Source: CAD feature listing. Evaluate the final solid. Frame: model axes, mm. Face numbers are marked on the shaded views. A direction names the side the tool comes from. Round coordinates to 2 decimals unless told otherwise and drop trailing zeros. Loops run counter-clockwise (first coordinate to the right, second up) from the corner with the lowest first, then second, coordinate; pieces in that order, holes last. Notation, with made-up numbers: (-30, 22.5) - (17, 22.5) arc R26 ccw to (17, 52.5) - close; hole circle Ø11 at (5.25, 45). An arc over 180 degrees is marked (long way). Use CSV: the item, a comma, the result in double quotes. Start each with the question number.
from build123d import *

# Parameters (mm, degrees)
BOSS_EXTRUDE1_DEPTH = 2
BOSS_EXTRUDE2_DEPTH = 3.2
SKETCH3_OUTSIDE_W   = 10.04
SKETCH3_OUTSIDE_H   = 5.89
CUT_EXTRUDE1_DEPTH  = 4.8
SKETCH4_W           = 1
SKETCH4_H           = 0.3
CUT_EXTRUDE3_DEPTH  = 2.3
CUT_EXTRUDE6_DEPTH  = 7.038418667
SKETCH6_W           = 0.5
SKETCH6_H           = 0.5
CUT_EXTRUDE7_DEPTH  = 2
SKETCH7_W           = 0.5
SKETCH7_H           = 0.8
CUT_EXTRUDE8_DEPTH  = 7
SKETCH8_W           = 6
SKETCH8_H           = 1
CUT_EXTRUDE9_DEPTH  = 0.5


with BuildPart() as part:
    # Sketch1 → Boss-Extrude1 (new body)
    with BuildSketch(Plane.XY):
        with BuildLine():
            Line((-2.7, 1.5), (2.7, 1.5))
            ThreePointArc((2.7, 1.5), (2.912132034, 1.412132034), (3, 1.2))
            Line((3, 1.2), (3, 0))
            Line((3, 0), (-3, 0))
            Line((-3, 0), (-3, 1.2))
            ThreePointArc((-3, 1.2), (-2.912132034, 1.412132034), (-2.7, 1.5))
        make_face()
    extrude(amount=BOSS_EXTRUDE1_DEPTH)

    # Sketch2 → Boss-Extrude2 (add, symmetric)
    with BuildSketch(Plane(origin=(0, 0, 0), x_dir=(0, 0, -1), z_dir=(1, 0, 0))):
        with BuildLine():
            Line((0, 2.25), (-4.2, 2.25))
            ThreePointArc((-4.2, 2.25), (-4.6, 1.85), (-4.2, 1.45))
            Line((-4.2, 1.45), (0, 1.45))
            Line((0, 1.45), (0, 2.25))
        make_face()
    extrude(amount=BOSS_EXTRUDE2_DEPTH, both=True)

    # Sketch3 outside → Cut-Extrude1 (cut)
    with BuildSketch(Plane.XY.offset(2)):
        with Locations((0, 1.125)):
            Rectangle(SKETCH3_OUTSIDE_W, SKETCH3_OUTSIDE_H)
        with BuildLine():
            Line((-2, 2.2), (2, 2.2))
            ThreePointArc((2, 2.2), (2.212132034, 2.112132034), (2.3, 1.9))
            Line((2.3, 1.9), (2.3, 1.1))
            Line((2.3, 1.1), (1.8, 0.6))
            Line((1.8, 0.6), (-1.8, 0.6))
            Line((-1.8, 0.6), (-2.3, 1.1))
            Line((-2.3, 1.1), (-2.3, 1.9))
            ThreePointArc((-2.3, 1.9), (-2.212132034, 2.112132034), (-2, 2.2))
        make_face(mode=Mode.SUBTRACT)
    extrude(amount=-CUT_EXTRUDE1_DEPTH, mode=Mode.SUBTRACT)

    # Sketch4 → Cut-Extrude3 (cut)
    with BuildSketch(Plane.XY):
        with Locations((0, 2.05)):
            Rectangle(SKETCH4_W, SKETCH4_H)
    extrude(amount=CUT_EXTRUDE3_DEPTH, mode=Mode.SUBTRACT)

    # Sketch5 → Cut-Extrude6 (cut, through all)
    with BuildSketch(Plane(origin=(0, 0, 0), x_dir=(1, 0, 0), z_dir=(0, 1, 0))):
        Polygon((-1.85, 0), (1.85, 0), (1.85, -1), (1.35, -1), (1.35, -0.7), (1.05, -0.7), (1.05, -1), (0.55, -1), (0.55, -0.7), (0.25, -0.7), (0.25, -1), (-0.25, -1), (-0.25, -0.7), (-0.55, -0.7), (-0.55, -1), (-1.05, -1), (-1.05, -0.7), (-1.35, -0.7), (-1.35, -1), (-1.85, -1), align=None)
    extrude(amount=CUT_EXTRUDE6_DEPTH, mode=Mode.SUBTRACT)

    # Sketch6 → Cut-Extrude7 (cut)
    with BuildSketch(Plane.XY.offset(2)):
        with Locations((1.6, 1.65)):
            Rectangle(SKETCH6_W, SKETCH6_H)
        with Locations((0.8, 1.65)):
            Rectangle(SKETCH6_W, SKETCH6_H)
        with Locations((0, 1.65)):
            Rectangle(SKETCH6_W, SKETCH6_H)
        with Locations((-0.8, 1.65)):
            Rectangle(SKETCH6_W, SKETCH6_H)
        with Locations((-1.6, 1.65)):
            Rectangle(SKETCH6_W, SKETCH6_H)
    extrude(amount=-CUT_EXTRUDE7_DEPTH, mode=Mode.SUBTRACT)

    # Sketch7 → Cut-Extrude8 (cut)
    with BuildSketch(Plane.XY):
        with Locations((1.6, 2)):
            Rectangle(SKETCH7_W, SKETCH7_H)
        with Locations((0.8, 2)):
            Rectangle(SKETCH7_W, SKETCH7_H)
        with Locations((0, 2)):
            Rectangle(SKETCH7_W, SKETCH7_H)
        with Locations((-0.8, 2)):
            Rectangle(SKETCH7_W, SKETCH7_H)
        with Locations((-1.6, 2)):
            Rectangle(SKETCH7_W, SKETCH7_H)
    extrude(amount=CUT_EXTRUDE8_DEPTH, mode=Mode.SUBTRACT)

    # Sketch8 → Cut-Extrude9 (cut)
    with BuildSketch(Plane(origin=(0, 0.6, 0), x_dir=(1, 0, 0), z_dir=(0, 1, 0))):
        with Locations((0, -0.5)):
            Rectangle(SKETCH8_W, SKETCH8_H)
    extrude(amount=CUT_EXTRUDE9_DEPTH, mode=Mode.SUBTRACT)


solid = part.part
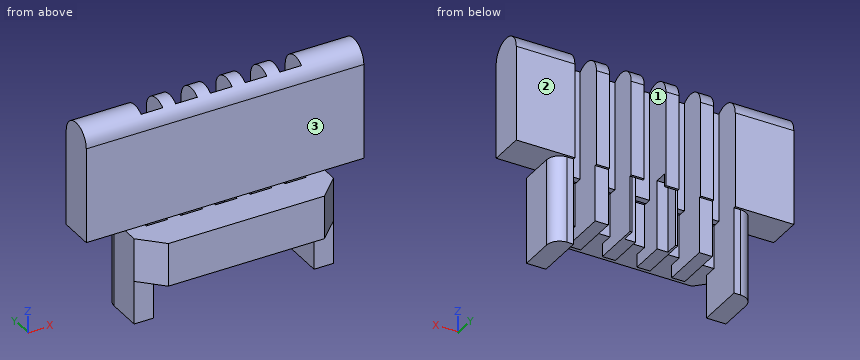
1. Section query A-A on z = 0.8. Give the number of separate pieces and of enclosed holes in the cut face, and give its area (3 significant figures).
2. Reachability of the marked faces 1, 2 and 3 from +Z, -Z, +X, -X, +Y, -Y: full face, straight path, thin tool, end or side. Return the list, or none.
3. Contact query for flat-ended pins moving along their axis: P1, Ø0.6, axis at x = -1.5, z = 1.5, coming from the +Y side; P2, Ø0.9, axis at y = 1.5, z = 1.5, coming from the +X side. Output: stop coordinate, or through.
4. Section query C-C on y = 1.75. Return the cut outline in (x, z), and give its area (3 significant figures).
5. Section query B-B on x = 0. Return the cut outline in (y, z).
6. Section query D-D on x = -1.25. Return the cut outline in (y, z).
7. Line query: line 1 along X through (y, z) = (1.65, 4.1); line 2 along X through (y, z) = (1.5, 0.55). Output: solid intervals per line, ascending.
Values:
1,separate pieces,"6"
1,enclosed holes,"0"
1,area,"2.12 mm^2"
2,face 1,"-Z, +Y"
2,face 2,"+Z, -Z, +X, -X, +Y"
2,face 3,"+Z, +X, -X, -Y"
3,P1,"stops at y = 2.2"
3,P2,"stops at x = 2.3"
4,outline,"(-3.2, 2) - (-2.3, 2) - (-2.3, 0) - (-1.85, 0) - (-1.85, 4.59) - (-3.2, 4.59) - close; (-1.35, 0.7) - (-1.05, 0.7) - (-1.05, 4.59) - (-1.35, 4.59) - close; (-0.55, 0.7) - (-0.25, 0.7) - (-0.25, 4.59) - (-0.55, 4.59) - close; (0.25, 0.7) - (0.55, 0.7) - (0.55, 4.59) - (0.25, 4.59) - close; (1.05, 0.7) - (1.35, 0.7) - (1.35, 4.59) - (1.05, 4.59) - close; (1.85, 0) - (2.3, 0) - (2.3, 2) - (3.2, 2) - (3.2, 4.59) - (1.85, 4.59) - close"
4,area,"13.5 mm^2"
5,outline,"(0.6, 1) - (1.4, 1) - (1.4, 2) - (0.6, 2) - close; (1.45, 2) - (1.6, 2) - (1.6, 4.51) arc R0.4 ccw to (1.45, 4.2) - close"
6,outline,"(0.6, 1) - (1.1, 1) - (1.1, 0.7) - (2.2, 0.7) - (2.2, 2) - (2.25, 2) - (2.25, 4.2) arc R0.4 ccw to (1.45, 4.2) - (1.45, 2) - (0.6, 2) - close"
7,line 1,"x = -3.2 to -1.85, -1.35 to -1.05, -0.55 to -0.25, 0.25 to 0.55, 1.05 to 1.35, 1.85 to 3.2"
7,line 2,"x = -2.3 to -1.85, 1.85 to 2.3"
